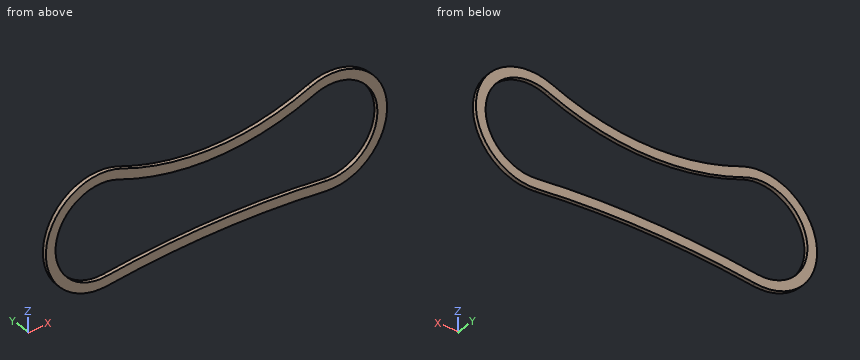
from build123d import *

# Parameters (mm, degrees)
F1_DEPTH = 20


with BuildPart() as f1:
    # F0 (on Front) → F1 (new body)
    with BuildSketch(Plane.XZ):
        with BuildLine():
            ThreePointArc((-575.276073, -283.535894), (-13.43211, -249.619942), (548.557665, -281.027318))
            ThreePointArc((548.557665, -281.027318), (863.797054, 42.135967), (472.103942, 266.606204))
            ThreePointArc((472.103942, 266.606204), (-14.367937, 169.627757), (-501.26791, 264.433483))
            ThreePointArc((-501.26791, 264.433483), (-891.955016, 38.216849), (-575.276073, -283.535894))
        make_face()
        with BuildLine():
            ThreePointArc((-581.179886, -233.885667), (-842.283064, 32.413932), (-518.471458, 217.444713))
            ThreePointArc((-518.471458, 217.444713), (-17.331035, 119.5998), (483.85336, 217.21923))
            ThreePointArc((483.85336, 217.21923), (491.242064, 220.413793), (498.735616, 223.354006))
            ThreePointArc((498.735616, 223.354006), (814.804212, 31.195097), (554.239766, -231.35123))
            ThreePointArc((554.239766, -231.35123), (-13.543718, -199.620066), (-581.179886, -233.885667))
        make_face(mode=Mode.SUBTRACT)
    extrude(amount=F1_DEPTH)


solid = f1.part
The listing builds one solid part. Answer for the finished solid, in the listing's coordinates (mm). Give positions to 0.01 mm unless a question says otherwise; leave off trailing zeros. Write each loop counter-clockwise with the first axis right and the second up, starting at its lowest first coordinate (ties: lowest second). Pieces come first, ordered by that corner, then holes. Notation, with made-up numbers: (44, 27.25) - (96, 27.25) arc R22 cw to (96, 37.25) - close; hole circle Ø9 at (46.5, -26). An arc over 180 degrees is marked (long way). One line per question, with ' | ' between items. Start each with the question number.
1. Section B-B, the plane y = -3 is taken. Determine the outline of the cut face in (x, z), then the cut area to 3 significant figures.
2. Straight lines are drawn through the part: line 1 (X direction, y = -7.5, z = 0); line 2 (Z direction, x = -5, y = -3.5); line 3 (Z direction, x = 6.5, y = -18.5). For each, find the intervals that lie inside material, in ascending order.
3. Section D-D, the plane z = 185 is taken. Determine the outline of the cut face in (x, y).
4. Section A-A, the plane z = 88.5 is taken. Determine the outline of the cut face in (x, y).
5. Section C-C, the plane x = 700.5 is taken. Determine the outline of the cut face in (y, z).
6. Given P1, Ø6, axis at y = -6.5, z = 197.5, coming from the -X side; P2, Ø1, axis at y = -9, z = 23, coming from the +X side, each flat-ended and moving along its own axis, determine where each tip first touches the part or whether it passes through.
Result:
1) outline: (-575.28, -283.54) arc R4850 cw to (548.56, -281.03) arc R285.53 ccw (long way) to (472.1, 266.61) arc R1283 cw to (-501.27, 264.43) arc R285.53 ccw (long way) to start; hole (-581.18, -233.89) arc R4900 cw to (554.24, -231.35) arc R235.53 ccw (long way) to (498.74, 223.35) arc R235.53 ccw to (483.85, 217.22) arc R1333.83 cw to (-518.47, 217.44) arc R235.53 ccw (long way) to start | area: 203,000 mm2
2) line 1: x = -894.52 to -844.52, 816.52 to 866.53 | line 2: z = -249.61 to -199.61, 119.65 to 169.68 | line 3: z = -249.62 to -199.62, 119.81 to 169.84
3) outline: (-826.49, -20) - (-754.77, -20) - (-754.77, 0) - (-826.49, 0) - close; (-429.57, -20) - (-215.26, -20) - (-215.26, 0) - (-429.57, 0) - close; (180.8, -20) - (395.51, -20) - (395.51, 0) - (180.8, 0) - close; (730.09, -20) - (800.73, -20) - (800.73, 0) - (730.09, 0) - close
4) outline: (-880.46, -20) - (-827.27, -20) - (-827.27, 0) - (-880.46, 0) - close; (800.34, -20) - (853.33, -20) - (853.33, 0) - (800.34, 0) - close
5) outline: (-20, -256.67) - (0, -256.67) - (0, -200.31) - (-20, -200.31) - close; (-20, 205.63) - (0, 205.63) - (0, 261.98) - (-20, 261.98) - close
6) P1: stops at x = -818.03 | P2: stops at x = 865.85
